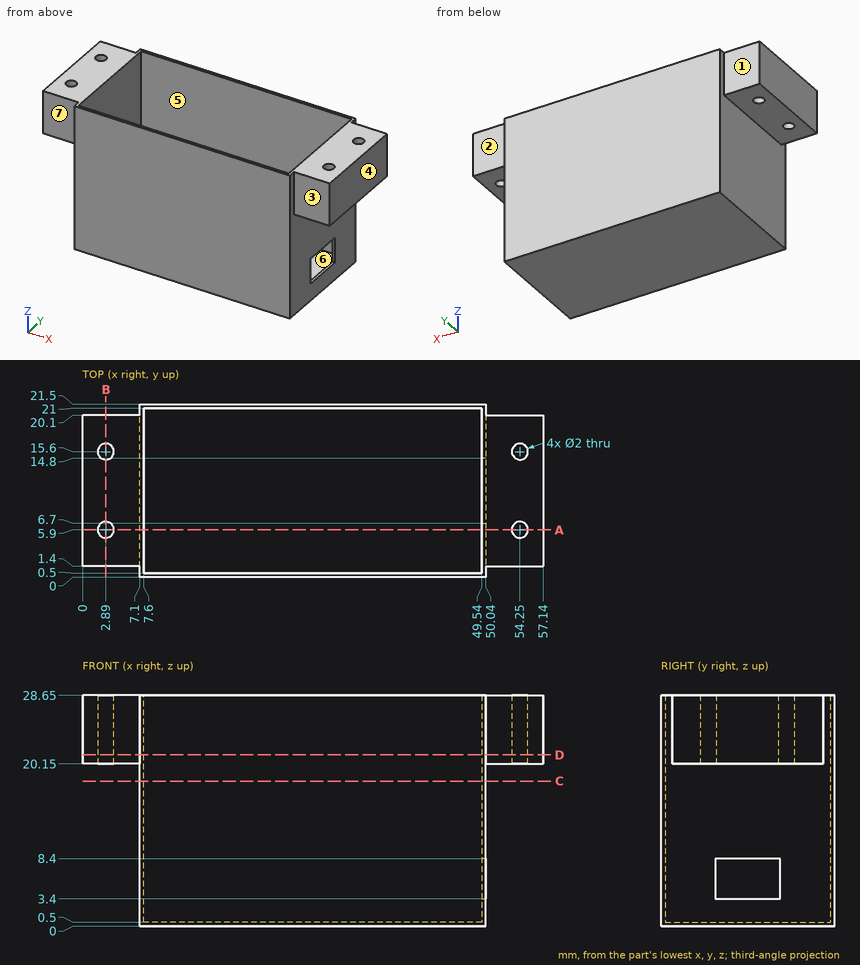
Input: dimensioned drawing with shaded views. Units: mm. Origin: part minimum x, y, z. A direction names the side the tool comes from. Coordinates: 2 decimals unless noted, no trailing zeros. Write each loop counter-clockwise with the first axis right and the second up, starting at its lowest first coordinate (ties: lowest second). Pieces come first, ordered by that corner, then holes. Notation, with made-up numbers: M 40,14.25 L 58,14.25 A7 ccw 58,19.25 Z; hole C 58.5,48.5 d8. An arc over 180 degrees is marked long. Use a Markdown table: item, result.
1) Section C-C, the plane z = 18. Output: boundary loops of the cut face in (x, y), then the cut area to 3 significant figures.
Conclusion:
| item | result |
|---|---|
| outline | M 7.1,0 L 50.04,0 L 50.04,21.5 L 7.1,21.5 Z; hole M 7.6,0.5 L 49.54,0.5 L 49.54,21 L 7.6,21 Z |
| area | 63.4 mm^2 |
2) Section B-B, the plane x = 2.89. Output: boundary loops of the cut face in (y, z).
Conclusion:
| item | result |
|---|---|
| outline | M 1.4,20.15 L 4.9,20.15 L 4.9,28.65 L 1.4,28.65 Z; M 6.9,20.15 L 14.6,20.15 L 14.6,28.65 L 6.9,28.65 Z; M 16.6,20.15 L 20.1,20.15 L 20.1,28.65 L 16.6,28.65 Z |
3) Mould query, pull axis X, two halves, no side actions, for the marked faces 4, 5, 6 and 7. Classes: pulls with the +X half, pulls with the -X half, needs draft (parallel to the pull), parting line crosses it, or undercut.
Conclusion:
| item | result |
|---|---|
| face 4 | pulls with the +X half |
| face 5 | undercut |
| face 6 | undercut |
| face 7 | needs draft |
4) Section A-A, the plane y = 5.9. Output: boundary loops of the cut face in (x, z), then the cut area to 3 significant figures.
Conclusion:
| item | result |
|---|---|
| outline | M 0,20.15 L 1.89,20.15 L 1.89,28.65 L 0,28.65 Z; M 3.89,20.15 L 7.1,20.15 L 7.1,0 L 50.04,0 L 50.04,20.15 L 53.25,20.15 L 53.25,28.65 L 49.54,28.65 L 49.54,0.5 L 7.6,0.5 L 7.6,28.65 L 3.89,28.65 Z; M 55.25,20.15 L 57.14,20.15 L 57.14,28.65 L 55.25,28.65 Z |
| area | 136 mm^2 |
5) Section D-D, the plane z = 21.25. Output: boundary loops of the cut face in (x, y), then the cut area to 3 significant figures.
Conclusion:
| item | result |
|---|---|
| outline | M 0,1.4 L 7.1,1.4 L 7.1,0 L 50.04,0 L 50.04,1.4 L 57.14,1.4 L 57.14,20.1 L 50.04,20.1 L 50.04,21.5 L 7.1,21.5 L 7.1,20.1 L 0,20.1 Z; hole C 2.89,5.9 d2; hole C 2.89,15.6 d2; hole M 7.6,0.5 L 49.54,0.5 L 49.54,21 L 7.6,21 Z; hole C 54.25,5.9 d2; hole C 54.25,15.6 d2 |
| area | 316 mm^2 |
6) Reachability of the marked faces 1, 2 and 3 from +Z, -Z, +X, -X, +Y, -Y: full face, straight path, thin tool, end or side. Return the list, or none.
Conclusion:
| item | result |
|---|---|
| face 1 | +Z, -Z, -X, +Y |
| face 2 | +Z, -Z, +X, +Y |
| face 3 | +Z, -Z, +X, -Y |
7) Ray query, L1, parallel to Y at x = 2.89, z = 24.75; L2, parallel to X at y = 5.9, z = 24; L3, parallel to Y at x = 45, z = 5. Return the intervals inside material, ascending.
Conclusion:
| item | result |
|---|---|
| L1 | y = 1.4 to 4.9, 6.9 to 14.6, 16.6 to 20.1 |
| L2 | x = 0 to 1.89, 3.89 to 7.6, 49.54 to 53.25, 55.25 to 57.14 |
| L3 | y = 0 to 0.5, 21 to 21.5 |
8) First-contact query: pin 1 Ø10 at (y, z) = (10, 13.5) entering from -X; pin 2 Ø1.6 at (x, y) = (2.89, 15.6) entering from +Z; pin 3 Ø3.5 at (x, y) = (2, 13) entering from -Z; pin 4 Ø2 at (x, y) = (10.5, 18) entering from +Z. Flat tips, straight axial feed; report the tip coordinate or a pass-through.
Conclusion:
| item | result |
|---|---|
| pin 1 | stops at x = 7.1 |
| pin 2 | passes through |
| pin 3 | stops at z = 20.15 |
| pin 4 | stops at z = 0.5 |
